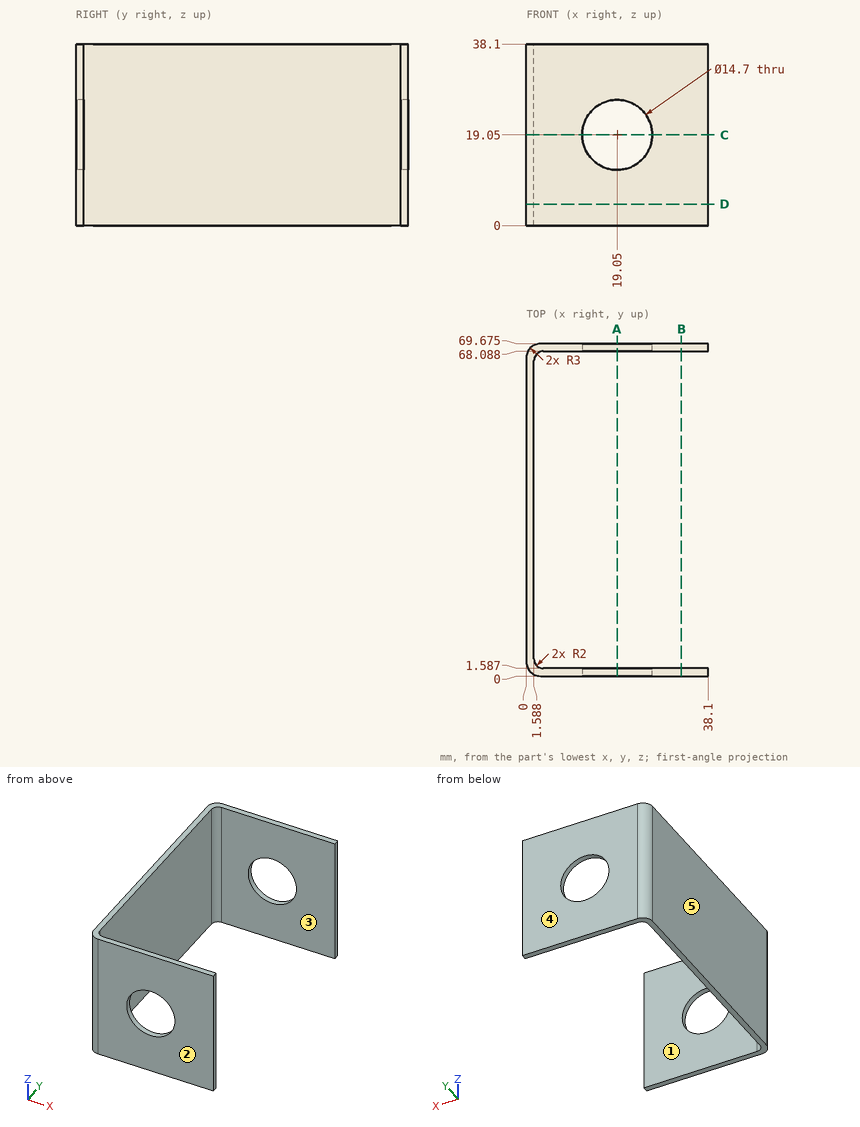
Drawing for the job (mm, zero at the part's lowest x, y, z). A direction names the side the tool comes from. Coordinates: 2 decimals unless noted, no trailing zeros. Order: outer loops, then holes, each group sorted by start corner. A loop starts at its lowest first (then second) coordinate and runs counter-clockwise, first axis right, second up. Notation, with made-up numbers: (22.5, 43.5) - (32.5, 43.5) arc R22 cw to (32.5, 51.5) - close; hole circle Ø2 at (-16, 18.25). An arc over 180 degrees is marked (long way). Use a Markdown table: item, result. Add a question column.
(1) Pull direction Y, two halves, no side cores. Call the marked faces 3, 4 and 5: +Y half, -Y half, draft (parallel to the pull), parting line (faces both ways), or undercut.
(2) Saw through at A-A (x = 19.05). Give the cut face in (y, z) (1 decimal).
(3) Flat gauge pins, fed straight in: pin 1 (8 mm diameter, centred on y = 8.5, z = 23, fed in from -X); pin 2 (10 mm diameter, centred on y = 53, z = 19, fed in from +X). Where does each tip first touch, or does it go through?
(4) Saw through at D-D (z = 4.5). Give the cut face in (x, y) (1 decimal).
(5) Drill centre lines: line 1 along Y through (x, z) = (35, 7) (1 decimal); line 2 along Z through (x, y) = (19.05, 0.95); line 3 along X through (y, z) = (62.5, 35.5). Where is each one in solid material? Low to high. Write a range as [from, to].
(6) Saw through at C-C (z = 19.05). Give the cut face in (x, y) (1 decimal).
(7) Saw through at B-B (x = 32.5). Give the cut face in (y, z) (1 decimal).
(8) Which spindle directions (+Z, -Z, +X, -X, +Y, -Y) get a long thin tool onto all of the face, cutting with end or side? Do the marked faces 1 and 2. Say none if no direction does.
Solved:
| question | item | result |
|---|---|---|
| 1 | face 3 | undercut |
| 1 | face 4 | +Y half |
| 1 | face 5 | draft |
| 2 | outline | (0, 0) - (1.6, 0) - (1.6, 11.7) - (0, 11.7) - close; (0, 26.4) - (1.6, 26.4) - (1.6, 38.1) - (0, 38.1) - close; (68.1, 0) - (69.7, 0) - (69.7, 11.7) - (68.1, 11.7) - close; (68.1, 26.4) - (69.7, 26.4) - (69.7, 38.1) - (68.1, 38.1) - close |
| 3 | pin 1 | stops at x = 0 |
| 3 | pin 2 | stops at x = 1.59 |
| 4 | outline | (0, 3) arc R3 ccw to (3, 0) - (38.1, 0) - (38.1, 1.6) - (3.6, 1.6) arc R2 cw to (1.6, 3.6) - (1.6, 66.1) arc R2 cw to (3.6, 68.1) - (38.1, 68.1) - (38.1, 69.7) - (3, 69.7) arc R3 ccw to (0, 66.7) - close |
| 5 | line 1 | y = [0, 1.6], [68.1, 69.7] |
| 5 | line 2 | z = [0, 11.7], [26.4, 38.1] |
| 5 | line 3 | x = [0, 1.59] |
| 6 | outline | (0, 3) arc R3 ccw to (3, 0) - (11.7, 0) - (11.7, 1.6) - (3.6, 1.6) arc R2 cw to (1.6, 3.6) - (1.6, 66.1) arc R2 cw to (3.6, 68.1) - (11.7, 68.1) - (11.7, 69.7) - (3, 69.7) arc R3 ccw to (0, 66.7) - close; (26.4, 0) - (38.1, 0) - (38.1, 1.6) - (26.4, 1.6) - close; (26.4, 68.1) - (38.1, 68.1) - (38.1, 69.7) - (26.4, 69.7) - close |
| 7 | outline | (0, 0) - (1.6, 0) - (1.6, 38.1) - (0, 38.1) - close; (68.1, 0) - (69.7, 0) - (69.7, 38.1) - (68.1, 38.1) - close |
| 8 | face 1 | +Z, -Z, +X |
| 8 | face 2 | +Z, -Z, +X, -X, -Y |
